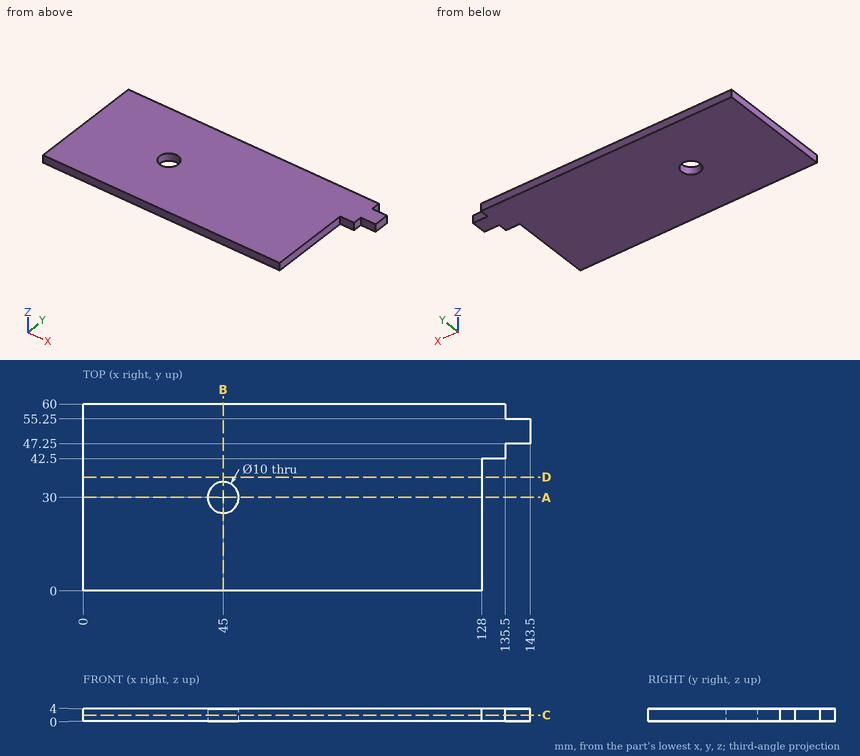
Answer from the drawing. Dimensions are ordinates in mm from the lowest x, y and z of the part. Round coordinates to 2 decimals unless told otherwise and drop trailing zeros. Loops run counter-clockwise (first coordinate to the right, second up) from the corner with the lowest first, then second, coordinate; pieces in that order, holes last. Notation, with made-up numbers: M 73.5,-19.5 L 78.5,-19.5 A25 ccw 78.5,19.5 Z; hole C 70,18.5 d3. An arc over 180 degrees is marked long. One line per question, with ' | ' between items. Start each with the question number.
(1) A cutting plane is placed at D-D on y = 36.5. Write down the section's boundary in (x, z), plus the area to 3 significant figures.
(2) Flat-ended cylindrical pins translate along their axes: pin 1 Ø1 at (y, z) = (38.5, 2.5) entering from +X; pin 2 Ø1.2 at (y, z) = (45.5, 2) entering from +X; pin 3 Ø2 at (x, z) = (132.5, 3) entering from -Y. Find the tip coordinate at first contact, or state that the pin passes through.
(3) Find the intervals of material crossed by line 1 (Y direction, x = 45, z = 2.7); line 2 (X direction, y = 16, z = 3.25); line 3 (X direction, y = 44.5, z = 2.3), in increasing order.
(4) A cutting plane is placed at A-A on y = 30. Write down the section's boundary in (x, z), plus the area to 3 significant figures.
(5) A cutting plane is placed at C-C on z = 2. Write down the section's boundary in (x, y).
(6) A cutting plane is placed at B-B on x = 45. Write down the section's boundary in (y, z).
Geometry check:
1) outline: M 0,0 L 128,0 L 128,4 L 0,4 Z | area: 512 mm²
2) pin 1: stops at x = 128 | pin 2: stops at x = 135.5 | pin 3: stops at y = 42.5
3) line 1: y = 0 to 25, 35 to 60 | line 2: x = 0 to 128 | line 3: x = 0 to 135.5
4) outline: M 0,0 L 40,0 L 40,4 L 0,4 Z; M 50,0 L 128,0 L 128,4 L 50,4 Z | area: 472 mm²
5) outline: M 0,0 L 128,0 L 128,42.5 L 135.5,42.5 L 135.5,47.25 L 143.5,47.25 L 143.5,55.25 L 135.5,55.25 L 135.5,60 L 0,60 Z; hole C 45,30 d10
6) outline: M 0,0 L 25,0 L 25,4 L 0,4 Z; M 35,0 L 60,0 L 60,4 L 35,4 Z
